Part model, mm, in its own coordinate system. Coordinates: 2 decimals unless noted, no trailing zeros. Order: outer loops, then holes, each group sorted by start corner. A loop starts at its lowest first (then second) coordinate and runs counter-clockwise, first axis right, second up.
from build123d import *

# Parameters (mm, degrees)
INNERCYLINDER_R     = 13.3223
INNERCYLINDER_DEPTH = 1200
OUTERCYLINDER_R     = 16.7005
OUTERCYLINDER_DEPTH = 1000


with BuildPart() as innercylinder:
    # InnerCylinder → InnerCylinder (new body)
    with BuildSketch(Plane.XY.offset(-100)):
        Circle(INNERCYLINDER_R)
    extrude(amount=INNERCYLINDER_DEPTH)


with BuildPart() as pipe:
    # OuterCylinder → OuterCylinder (new body)
    with BuildSketch(Plane.XY):
        Circle(OUTERCYLINDER_R)
    extrude(amount=OUTERCYLINDER_DEPTH)

    # Pipe: cut InnerCylinder
    add(innercylinder.part, mode=Mode.SUBTRACT)


solid = pipe.part
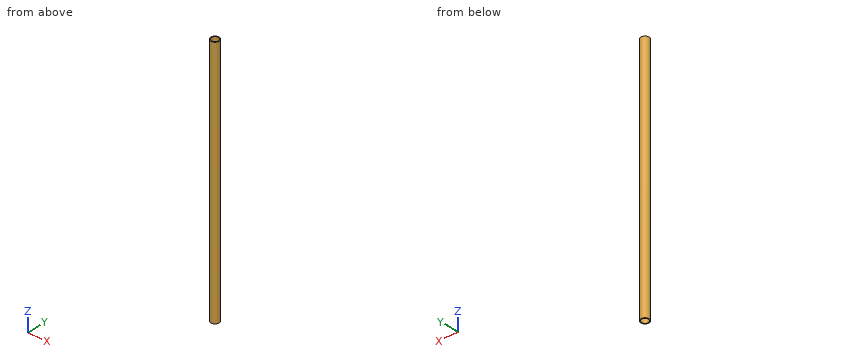
Q1. Wall check: line 1 along Y through (x, z) = (0, 732); line 2 along Y through (x, z) = (-2, 447); line 3 along X through (y, z) = (-1, 146). Give the ranges that are in metal, low to high.
Results list:
line 1: y = -16.7 to -13.32, 13.32 to 16.7
line 2: y = -16.58 to -13.17, 13.17 to 16.58
line 3: x = -16.67 to -13.28, 13.28 to 16.67
Q2. Pin check, flat tips, straight feed: pin 1 Ø8 at (y, z) = (-9.5, 865.5) entering from +X; pin 2 Ø2 at (x, z) = (-9.5, 106.5) entering from -Y; pin 3 Ø2 at (x, y) = (-12, 3) entering from -Z; pin 4 Ø5 at (x, z) = (3, 351) entering from +Y. Stop position of each tip, or through.
Results list:
pin 1: stops at x = 15.77
pin 2: stops at y = -14.38
pin 3: stops at z = 0
pin 4: stops at y = 16.69
Q3. Cut at C-C on z = 233.5. Write the cut outline in (x, y).
Results list:
outline: circle Ø33.4 at (0, 0); hole circle Ø26.64 at (0, 0)
Q4. Cut at A-A on x = 0. Write the cut outline in (y, z), and give its area (3 significant figures).
Results list:
outline: (-16.7, 0) - (-13.32, 0) - (-13.32, 1000) - (-16.7, 1000) - close; (13.32, 0) - (16.7, 0) - (16.7, 1000) - (13.32, 1000) - close
area: 6,760 mm2
